from build123d import *

# Parameters (mm, degrees)
SKETCH_1_R      = 1.5
SKETCH_1_R_2    = 3
EXTRUDE_1_DEPTH = 5


with BuildPart() as part:
    # 스케치1 → 보스-돌출1 (new body)
    with BuildSketch(Plane.XY):
        Polygon((0, 10.1), (0, 0.1), (140, 0.1), (140, 10.1), (140, 22.1), (0, 22.1), align=None)
        with Locations((40, 20.1)):
            Circle(SKETCH_1_R, mode=Mode.SUBTRACT)
        with Locations((70.5, 10.1)):
            Circle(SKETCH_1_R_2, mode=Mode.SUBTRACT)
        with Locations((100.5, 10.1)):
            Circle(SKETCH_1_R_2, mode=Mode.SUBTRACT)
        with Locations((130.5, 10.1)):
            Circle(SKETCH_1_R_2, mode=Mode.SUBTRACT)
        with Locations((9.5, 10.1)):
            Circle(SKETCH_1_R_2, mode=Mode.SUBTRACT)
        with BuildLine():
            Line((32.5, 10.1), (32.5, 10.6))
            ThreePointArc((32.5, 10.6), (40, 18.1), (47.5, 10.6))
            Line((47.5, 10.6), (47.5, 10.1))
            Line((47.5, 10.1), (47.5, 9.6))
            ThreePointArc((47.5, 9.6), (40, 2.1), (32.5, 9.6))
            Line((32.5, 9.6), (32.5, 10.1))
        make_face(mode=Mode.SUBTRACT)
        with BuildLine():
            Line((31.428932188, 3.028932188), (31.428932188, 3.528932188))
            ThreePointArc((31.428932188, 3.528932188), (32.928932188, 5.028932188), (34.428932188, 3.528932188))
            Line((34.428932188, 3.528932188), (34.428932188, 3.028932188))
            Line((34.428932188, 3.028932188), (34.428932188, 2.528932188))
            ThreePointArc((34.428932188, 2.528932188), (32.928932188, 1.028932188), (31.428932188, 2.528932188))
            Line((31.428932188, 2.528932188), (31.428932188, 3.028932188))
        make_face(mode=Mode.SUBTRACT)
        with BuildLine():
            Line((28.5, 10.1), (28.5, 10.6))
            ThreePointArc((28.5, 10.6), (30, 12.1), (31.5, 10.6))
            Line((31.5, 10.6), (31.5, 10.1))
            Line((31.5, 10.1), (31.5, 9.6))
            ThreePointArc((31.5, 9.6), (30, 8.1), (28.5, 9.6))
            Line((28.5, 9.6), (28.5, 10.1))
        make_face(mode=Mode.SUBTRACT)
        with BuildLine():
            Line((31.428932188, 17.171067812), (31.428932188, 17.671067812))
            ThreePointArc((31.428932188, 17.671067812), (32.928932188, 19.171067812), (34.428932188, 17.671067812))
            Line((34.428932188, 17.671067812), (34.428932188, 17.171067812))
            Line((34.428932188, 17.171067812), (34.428932188, 16.671067812))
            ThreePointArc((34.428932188, 16.671067812), (32.928932188, 15.171067812), (31.428932188, 16.671067812))
            Line((31.428932188, 16.671067812), (31.428932188, 17.171067812))
        make_face(mode=Mode.SUBTRACT)
        with BuildLine():
            Line((45.571067812, 17.171067812), (45.571067812, 16.671067812))
            ThreePointArc((45.571067812, 16.671067812), (47.071067812, 15.171067812), (48.571067812, 16.671067812))
            Line((48.571067812, 16.671067812), (48.571067812, 17.171067812))
            Line((48.571067812, 17.171067812), (48.571067812, 17.671067812))
            ThreePointArc((48.571067812, 17.671067812), (47.071067812, 19.171067812), (45.571067812, 17.671067812))
            Line((45.571067812, 17.671067812), (45.571067812, 17.171067812))
        make_face(mode=Mode.SUBTRACT)
        with BuildLine():
            Line((51.5, 10.1), (51.5, 9.6))
            ThreePointArc((51.5, 9.6), (50, 8.1), (48.5, 9.6))
            Line((48.5, 9.6), (48.5, 10.1))
            Line((48.5, 10.1), (48.5, 10.6))
            ThreePointArc((48.5, 10.6), (50, 12.1), (51.5, 10.6))
            Line((51.5, 10.6), (51.5, 10.1))
        make_face(mode=Mode.SUBTRACT)
        with BuildLine():
            Line((48.571067812, 3.028932188), (48.571067812, 3.528932188))
            ThreePointArc((48.571067812, 3.528932188), (47.071067812, 5.028932188), (45.571067812, 3.528932188))
            Line((45.571067812, 3.528932188), (45.571067812, 3.028932188))
            Line((45.571067812, 3.028932188), (45.571067812, 2.528932188))
            ThreePointArc((45.571067812, 2.528932188), (47.071067812, 1.028932188), (48.571067812, 2.528932188))
            Line((48.571067812, 2.528932188), (48.571067812, 3.028932188))
        make_face(mode=Mode.SUBTRACT)
    extrude(amount=EXTRUDE_1_DEPTH)


solid = part.part
Here's how the part is built. I have some questions about the finished solid (model axes, mm). A direction names the side the tool comes from. Give positions to 0.01 mm unless a question says otherwise; leave off trailing zeros. Loops run counter-clockwise (first coordinate to the right, second up) from the corner with the lowest first, then second, coordinate; pieces in that order, holes last. Notation, with made-up numbers: (-15, 14) -> (12, 14) arc R15 ccw to (12, 28) -> close; hole circle Ø8 at (17, 27). An arc over 180 degrees is marked (long way). One line per item, written item: value.
Q1. Suppose I cut it at A-A on x = 50. Please give me the cut outline in (y, z).
Answers follow:
outline: (0.1, 0) -> (8.1, 0) -> (8.1, 5) -> (0.1, 5) -> close; (12.1, 0) -> (22.1, 0) -> (22.1, 5) -> (12.1, 5) -> close
Q2. I'm going to push flat-ended pins straight in: pin 1 Ø5.5 at (x, y) = (70.5, 10.1) entering from -Z; pin 2 Ø0.5 at (y, z) = (10, 2.5) entering from -X. Where does each tip first touch, or does it pass through?
Answers follow:
pin 1: through
pin 2: x = 0
Q3. Suppose I cut it at B-B on x = 130.5. Please give me the cut outline in (y, z), then the cut area to 3 significant figures.
Answers follow:
outline: (0.1, 0) -> (7.1, 0) -> (7.1, 5) -> (0.1, 5) -> close; (13.1, 0) -> (22.1, 0) -> (22.1, 5) -> (13.1, 5) -> close
area: 80.0 mm^2
Q4. Suppose I cut it at C-C on z = 3.15. State how many separate pieces and enclosed holes the cut face has, then the cut area to 3 significant figures.
Answers follow:
separate pieces: 1
enclosed holes: 12
area: 2,710 mm^2
Q5. If I drill on line 1 along Y through (x, z) = (40, 2.8); line 2 along X through (y, z) = (18.5, 0.75); line 3 along Y through (x, z) = (130.5, 3.6), over which ranges is the centre line in solid material (lowest first)?
Answers follow:
line 1: 0.1 to 2.1, 18.1 to 18.6, 21.6 to 22.1
line 2: 0 to 31.68, 34.18 to 45.82, 48.32 to 140
line 3: 0.1 to 7.1, 13.1 to 22.1
Q6. We'd pull the mould along Y, two halves only. Please class faces 1 (the face through (140, 11, 2)), 2 (the face through (71, 22.1, 2)), 3 (the face through (11.11, 12.63, 2.46)): pulls with the +Y half, pulls with the -Y half, needs draft (parallel to the pull), parting line crosses it, or undercut.
Answers follow:
face 1: needs draft
face 2: pulls with the +Y half
face 3: undercut
Q7. On a 3-axis mill with a long thin cutter (end or side, diameter ignored), from which of +Z, -Z, +X, -X, +Y, -Y can I reach the whole of each face in a straight line? I mean faces 4 (the face through (69, 14, 5)), 5 (the face through (50, 12.1, 2.5)). Say none if no direction works.
Answers follow:
face 4: +Z, +X, -X, +Y, -Y
face 5: +Z, -Z
